```python
from build123d import *

# Parameters (mm, degrees)
CUT_EXTRUDE1_DEPTH = 6.35
CHAMFER1_SIZE      = 1.9812
CHAMFER2_SIZE      = 0.762


with BuildPart() as part:
    # Sketch1 → Base-Revolve (revolve)
    with BuildSketch(Plane.XY, mode=Mode.PRIVATE) as base_revolve_sk:
        Polygon((7.9502, 0), (11.9126, 0), (11.9126, 15.875), (0, 15.875), (0, -38.1), (7.9502, -38.1), align=None)
    revolve(base_revolve_sk.sketch.rotate(Axis((0, 0, 0), (0, 1, 0)), 90), axis=Axis((0, 0, 0), (0, 1, 0)))

    # Sketch2 → Cut-Extrude1 (cut)
    with BuildSketch(Plane(origin=(0, 15.875, 0), x_dir=(-1, 0, 0), z_dir=(0, 1, 0))):
        Polygon((3.666174209, -6.35), (-3.666174209, -6.35), (-7.332348419, 0), (-3.666174209, 6.35), (3.666174209, 6.35), (7.332348419, 0), align=None)
    extrude(amount=-CUT_EXTRUDE1_DEPTH, mode=Mode.SUBTRACT)

    # Chamfer1
    chamfer1_edges = [part.edges().sort_by_distance(p)[0] for p in [
        (0, 15.875, 11.9126),
    ]]
    chamfer(chamfer1_edges, length=CHAMFER1_SIZE)

    # Chamfer2
    chamfer2_edges = [part.edges().sort_by_distance(p)[0] for p in [
        (0, -38.1, 7.9502),
    ]]
    chamfer(chamfer2_edges, length=CHAMFER2_SIZE)


solid = part.part
```
The listing builds one solid part. Answer for the finished solid, in the listing's coordinates (mm). A direction names the side the tool comes from. Give positions to 0.01 mm unless a question says otherwise; leave off trailing zeros. Order: outer loops, then holes, each group sorted by start corner. A loop starts at its lowest first (then second) coordinate and runs counter-clockwise, first axis right, second up.
Item 1: Given pin 1 Ø1 at (x, z) = (-2, -6) entering from +Y (3 decimals); pin 2 Ø6.5 at (x, z) = (2.5, -1) entering from +Y (3 decimals); pin 3 Ø3 at (y, z) = (7.5, 7.5) entering from +X; pin 4 Ø5 at (x, y) = (4.5, -13.5) entering from -Z, each flat-ended and moving along its own axis, determine where each tip first touches the part or whether it passes through.
From the geometry:
pin 1: stops at y = 15.875
pin 2: stops at y = 9.525
pin 3: stops at x = 10.29
pin 4: stops at z = -7.69
Item 2: The part is cut by section A-A, the plane x = 0. Give the vertices of the cut face in (y, z) (3 decimals), and give its area (3 significant figures).
From the geometry:
outline: (-38.1, -7.188) - (-37.338, -7.95) - (0, -7.95) - (0, -11.913) - (13.894, -11.913) - (15.875, -9.931) - (15.875, -6.35) - (9.525, -6.35) - (9.525, 6.35) - (15.875, 6.35) - (15.875, 9.931) - (13.894, 11.913) - (0, 11.913) - (0, 7.95) - (-37.338, 7.95) - (-38.1, 7.188) - close
area: 899 mm2
Item 3: The part is cut by section B-B, the plane y = -10.5. Give the vertices of the cut face in (x, z), and give its area (3 significant figures).
From the geometry:
outline: circle Ø15.9 at (0, 0)
area: 199 mm2
Item 4: For a pull along X with two mould halves and no side action, classify faces 1 (the face through (5.474, 12.744, -3.219)), 2 (the face through (7.25, 7.04, 9.45)), 3 (the face through (0, -38.1, 0)) as pulls with the +X half, pulls with the -X half, needs draft (parallel to the pull), parting line crosses it, or undercut.
From the geometry:
face 1: undercut
face 2: parting line crosses it
face 3: needs draft
Item 5: Find the intervals of material crossed by probe 1 along Y at (x, z) = (-4.25, -4.25) (3 decimals); probe 2 along Z at (x, y) = (4.5, 11); probe 3 along Y at (x, z) = (-7.5, -5.75) (3 decimals), in increasing order.
From the geometry:
probe 1: y = -38.1 to 9.525
probe 2: z = -11.03 to -4.91, 4.91 to 11.03
probe 3: y = 0 to 15.875
Item 6: Which of the six approach directions +Z, -Z, +X, -X, +Y, -Y give full straight-line access (tool end or side, diameter ignored) to faces 4 (the face through (8, 0, 2)), 5 (the face through (-0.1, 15.875, -6.5)), 6 (the face through (0, 13, -6.35))?
From the geometry:
face 4: -Y
face 5: +Z, -Z, +X, -X, +Y
face 6: +Y
Item 7: The part is cut by section C-C, the plane y = 9. Give the vertices of the cut face in (x, z).
From the geometry:
outline: circle Ø23.83 at (0, 0)
